Part print with two shaded views. Sizes in mm from the minimum x, y, z corner. A direction names the side the tool comes from. Round coordinates to 2 decimals unless told otherwise and drop trailing zeros. Write each loop counter-clockwise with the first axis right and the second up, starting at its lowest first coordinate (ties: lowest second). Pieces come first, ordered by that corner, then holes. Notation, with made-up numbers: (21.5, 49.5) -> (60.5, 49.5) arc R23 cw to (60.5, 57.5) -> close; hole circle Ø6 at (20, -11). An arc over 180 degrees is marked (long way). Put each result on its own line as item: value. Start each with the question number.
1. Flat gauge pins, fed straight in: P1, Ø4, axis at x = 47, z = 5.5, coming from the -Y side; P2, Ø4, axis at y = 50.5, z = 4.5, coming from the +X side; P3, Ø2, axis at y = 44.5, z = 3.5, coming from the +X side (1 decimal). Where does each tip first touch, or does it go through?
2. Pull direction Y, two halves, no side cores. Call the marked faces 3, 4 and 5: pulls with the +Y half, pulls with the -Y half, needs draft (parallel to the pull), parting line crosses it, or undercut.
3. Saw through at A-A on x = 31.75. List the corners of the cut face in (y, z).
4. Drill centre lines: line 1 (Y direction, x = 31.75, z = 1.45); line 2 (Y direction, x = 32, z = 6.25) (1 decimal); line 3 (Z direction, x = 30, y = 40). Where is each one in solid material? Low to high. Write a range as from..to.
5. Saw through at C-C on z = 6.75. State how many separate pieces and enclosed holes the cut face has, and give its area (3 significant figures).
6. Saw through at D-D on x = 23. List the corners of the cut face in (y, z).
7. 3-axis set-ups, long thin cutter, end or side, ignore diameter. For the marked faces 1 and 2: which of +Z, -Z, +X, -X, +Y, -Y reach the whole face in a straight line?
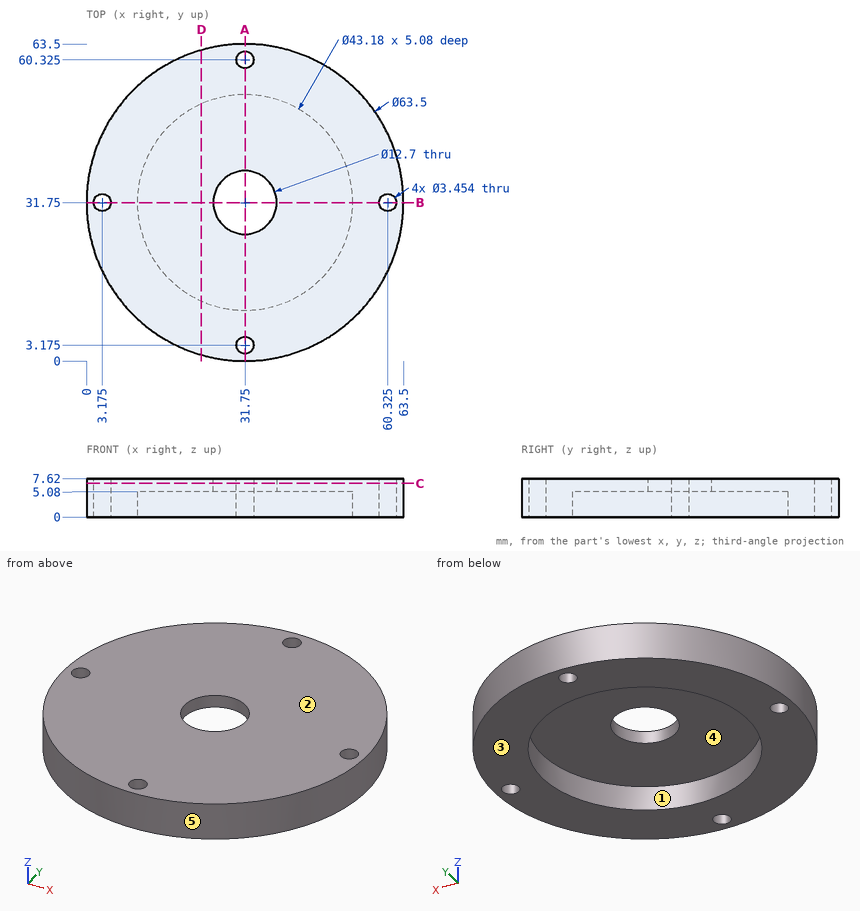
Return value:
1. P1: stops at y = 2.9
1. P2: stops at x = 58.72
1. P3: stops at x = 61.2
2. face 3: needs draft
2. face 4: undercut
2. face 5: parting line crosses it
3. outline: (0, 0) -> (1.45, 0) -> (1.45, 7.62) -> (0, 7.62) -> close; (4.9, 0) -> (10.16, 0) -> (10.16, 5.08) -> (25.4, 5.08) -> (25.4, 7.62) -> (4.9, 7.62) -> close; (38.1, 5.08) -> (53.34, 5.08) -> (53.34, 0) -> (58.6, 0) -> (58.6, 7.62) -> (38.1, 7.62) -> close; (62.05, 0) -> (63.5, 0) -> (63.5, 7.62) -> (62.05, 7.62) -> close
4. line 1: y = 0..1.45, 4.9..10.16, 53.34..58.6, 62.05..63.5
4. line 2: y = 0..1.5, 4.9..25.4, 38.1..58.6, 62..63.5
4. line 3: z = 5.08..7.62
5. separate pieces: 1
5. enclosed holes: 5
5. area: 3,000 mm^2
6. outline: (1.23, 0) -> (12.01, 0) -> (12.01, 5.08) -> (51.49, 5.08) -> (51.49, 0) -> (62.27, 0) -> (62.27, 7.62) -> (1.23, 7.62) -> close
7. face 1: -Z
7. face 2: +Z, +X, -X, +Y, -Y
